Drawing for the job (mm, zero at the part's lowest x, y, z). Give positions to 0.01 mm unless a question says otherwise; leave off trailing zeros. Write each loop counter-clockwise with the first axis right and the second up, starting at its lowest first coordinate (ties: lowest second). Pieces come first, ordered by that corner, then holes.
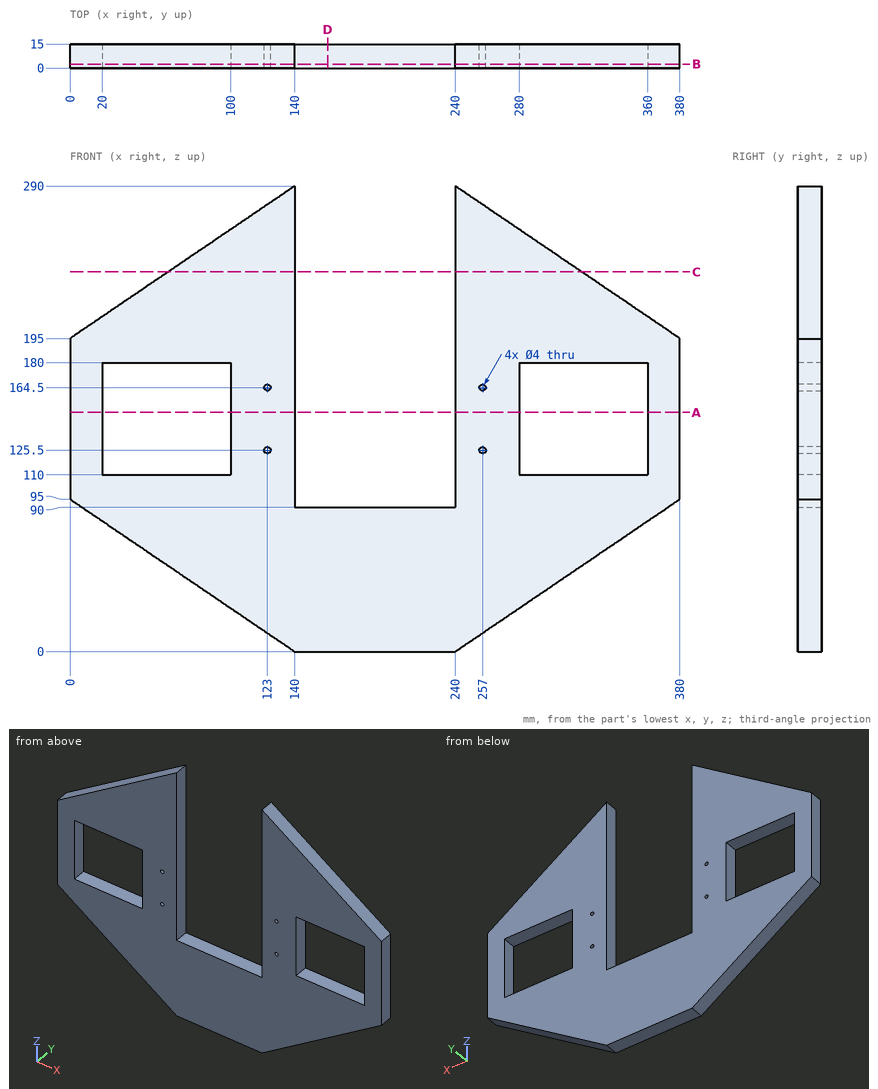
1. Slice it at D-D, the plane x = 160.5. Write the cut outline in (y, z).
Calculated:
outline: (0, 0) - (15, 0) - (15, 90) - (0, 90) - close
2. Slice it at A-A, the plane z = 149. Write the cut outline in (x, y), and give its area (3 significant figures).
Calculated:
outline: (0, 0) - (20, 0) - (20, 15) - (0, 15) - close; (100, 0) - (140, 0) - (140, 15) - (100, 15) - close; (240, 0) - (280, 0) - (280, 15) - (240, 15) - close; (360, 0) - (380, 0) - (380, 15) - (360, 15) - close
area: 1,800 mm2
3. Probe probe 1 along X at (y, z) = (5.5, 164.5); probe 2 along X at (y, z) = (12.5, 119.5); probe 3 along Z at (x, y) = (257, 9). List the from-to ranges inside material, lowest first.
Calculated:
probe 1: x = 0 to 20, 100 to 121, 125 to 140, 240 to 255, 259 to 280, 360 to 380
probe 2: x = 0 to 20, 100 to 140, 240 to 280, 360 to 380
probe 3: z = 11.54 to 123.5, 127.5 to 162.5, 166.5 to 278.46
4. Slice it at B-B, the plane y = 2.5. Write the cut outline in (x, z).
Calculated:
outline: (0, 95) - (140, 0) - (240, 0) - (380, 95) - (380, 195) - (240, 290) - (240, 90) - (140, 90) - (140, 290) - (0, 195) - close; hole (20, 110) - (100, 110) - (100, 180) - (20, 180) - close; hole circle Ø4 at (123, 125.5); hole circle Ø4 at (123, 164.5); hole circle Ø4 at (257, 125.5); hole circle Ø4 at (257, 164.5); hole (280, 110) - (360, 110) - (360, 180) - (280, 180) - close
5. Slice it at C-C, the plane z = 236.5. Write the cut outline in (x, y).
Calculated:
outline: (61.16, 0) - (140, 0) - (140, 15) - (61.16, 15) - close; (240, 0) - (318.84, 0) - (318.84, 15) - (240, 15) - close
6. Pin check, flat tips, straight feed: P1, Ø7.5, axis at y = 11, z = 223.5, coming from the -X side; P2, Ø6, axis at x = 246.5, y = 12, coming from the -Z side (3 decimals); P3, Ø4.5, axis at x = 56, y = 8.5, coming from the +Z side; P4, Ø5, axis at x = 257, z = 164.5, coming from the -Y side. Stop position of each tip, or through.
Calculated:
P1: stops at x = 36.47
P2: stops at z = 2.375
P3: stops at z = 234.53
P4: stops at y = 0
